Input: dimensioned drawing with shaded views. Units: mm. Origin: part minimum x, y, z. Give positions to 0.01 mm unless a question says otherwise; leave off trailing zeros. Write each loop counter-clockwise with the first axis right and the second up, starting at its lowest first coordinate (ties: lowest second). Pieces come first, ordered by that corner, then holes.
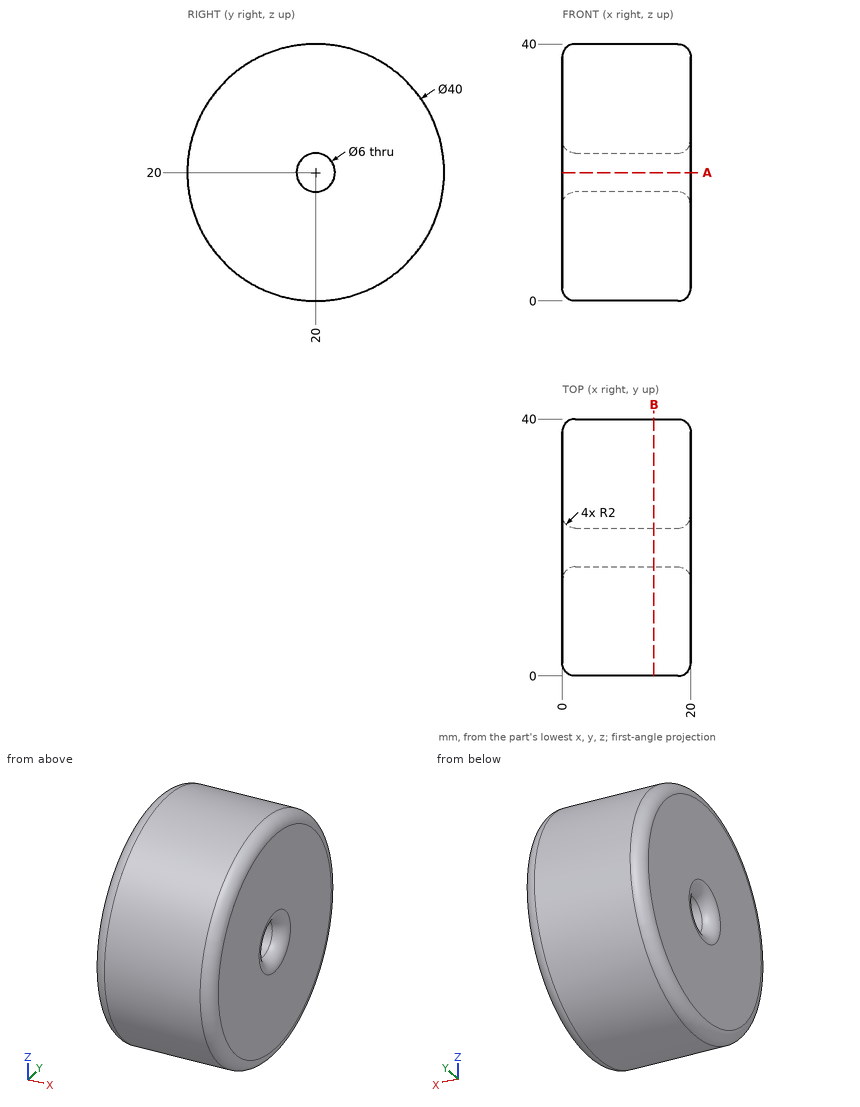
Item 1: Section B-B (x = 14.25). Return loops of the section in (y, z), and give its area (3 significant figures).
Item 2: Section A-A (z = 20). Return loops of the section in (x, y), and give its area (3 significant figures).
Item 3: Ray query, line 1 (Y direction, x = 1.75, z = 18); line 2 (X direction, y = 24.5, z = 22); line 3 (Y direction, x = 8.25, z = 19.5). Return the intervals inside material, ascending.
Item 4: Pin query (flat end, axial travel): pin 1 (8 mm diameter, centred on x = 10, y = 27.5, fed in from +Z); pin 2 (2 mm diameter, centred on x = 9.5, y = 11, fed in from +Z); pin 3 (12 mm diameter, centred on x = 7.5, y = 15, fed in from +Z). Return the tip coordinate at first contact, or that it passes through.
Solved:
1. outline: circle Ø40 at (20, 20); hole circle Ø6 at (20, 20)
1. area: 1,230 mm2
2. outline: (0, 2) arc R2 ccw to (2, 0) - (18, 0) arc R2 ccw to (20, 2) - (20, 15) arc R2 ccw to (18, 17) - (2, 17) arc R2 ccw to (0, 15) - close; (0, 25) arc R2 ccw to (2, 23) - (18, 23) arc R2 ccw to (20, 25) - (20, 38) arc R2 ccw to (18, 40) - (2, 40) arc R2 ccw to (0, 38) - close
2. area: 673 mm2
3. line 1: y = 0.12 to 17.74, 22.26 to 39.88
3. line 2: x = 0 to 20
3. line 3: y = 0.01 to 17.04, 22.96 to 39.99
4. pin 1: stops at z = 39.69
4. pin 2: stops at z = 38.33
4. pin 3: stops at z = 40
